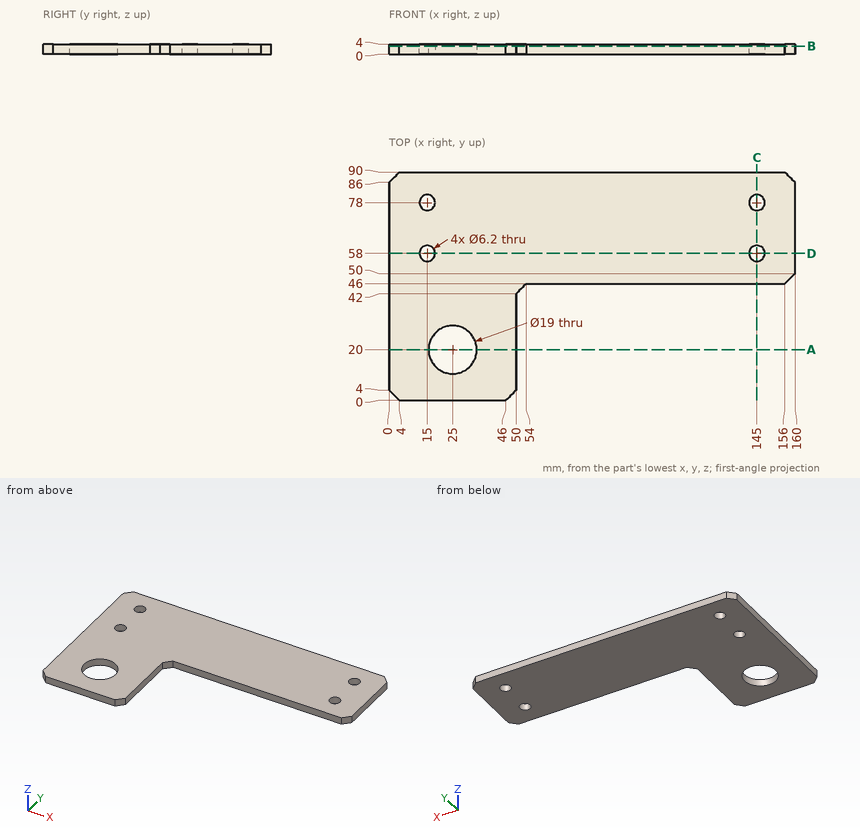
Answer from the drawing. Dimensions are ordinates in mm from the lowest x, y and z of the part. Give positions to 0.01 mm unless a question says otherwise; leave off trailing zeros. Order: outer loops, then holes, each group sorted by start corner. A loop starts at its lowest first (then second) coordinate and runs counter-clockwise, first axis right, second up. Notation, with made-up numbers: (-38.5, 18) -> (-13.5, 18) arc R22 cw to (-13.5, 47) -> close; hole circle Ø7 at (20, 15). An arc over 180 degrees is marked (long way). Answer as a JSON object with one key per item and string values. Group by question number.
1. Section D-D on y = 58 is taken. Determine the outline of the cut face in (x, z).
2. Section C-C on x = 145 is taken. Determine the outline of the cut face in (y, z), plus the area to 3 significant figures.
3. Consider line 1 along Y through (x, z) = (15, 2.25); line 2 along Y through (x, z) = (25, 1.3); line 3 along Y through (x, z) = (145, 2.2). Determine where each line is inside the solid, lowest interval first. Write a range as [from, to].
4. Section B-B on z = 3.15 is taken. Determine the outline of the cut face in (x, y).
5. Flat-ended cylindrical pins translate along their axes: pin 1 Ø5 at (x, y) = (15, 78) entering from +Z; pin 2 Ø1.5 at (y, z) = (43, 2.5) entering from +X; pin 3 Ø1 at (x, z) = (82, 0.5) entering from -Y. Find the tip coordinate at first contact, or state that the pin passes through.
6. Section A-A on y = 20 is taken. Determine the outline of the cut face in (x, z), plus the area to 3 significant figures.
Result sheet:
{
 "1": {"outline": "(0, 0) -> (11.9, 0) -> (11.9, 4) -> (0, 4) -> close; (18.1, 0) -> (141.9, 0) -> (141.9, 4) -> (18.1, 4) -> close; (148.1, 0) -> (160, 0) -> (160, 4) -> (148.1, 4) -> close"},
 "2": {"outline": "(46, 0) -> (54.9, 0) -> (54.9, 4) -> (46, 4) -> close; (61.1, 0) -> (74.9, 0) -> (74.9, 4) -> (61.1, 4) -> close; (81.1, 0) -> (90, 0) -> (90, 4) -> (81.1, 4) -> close", "area": "126 mm^2"},
 "3": {"line 1": "y = [0, 54.9], [61.1, 74.9], [81.1, 90]", "line 2": "y = [0, 10.5], [29.5, 90]", "line 3": "y = [46, 54.9], [61.1, 74.9], [81.1, 90]"},
 "4": {"outline": "(0, 4) -> (4, 0) -> (46, 0) -> (50, 4) -> (50, 42) -> (54, 46) -> (156, 46) -> (160, 50) -> (160, 86) -> (156, 90) -> (4, 90) -> (0, 86) -> close; hole circle Ø6.2 at (15, 58); hole circle Ø6.2 at (15, 78); hole circle Ø19 at (25, 20); hole circle Ø6.2 at (145, 58); hole circle Ø6.2 at (145, 78)"},
 "5": {"pin 1": "passes through", "pin 2": "stops at x = 51.75", "pin 3": "stops at y = 46"},
 "6": {"outline": "(0, 0) -> (15.5, 0) -> (15.5, 4) -> (0, 4) -> close; (34.5, 0) -> (50, 0) -> (50, 4) -> (34.5, 4) -> close", "area": "124 mm^2"}
}
